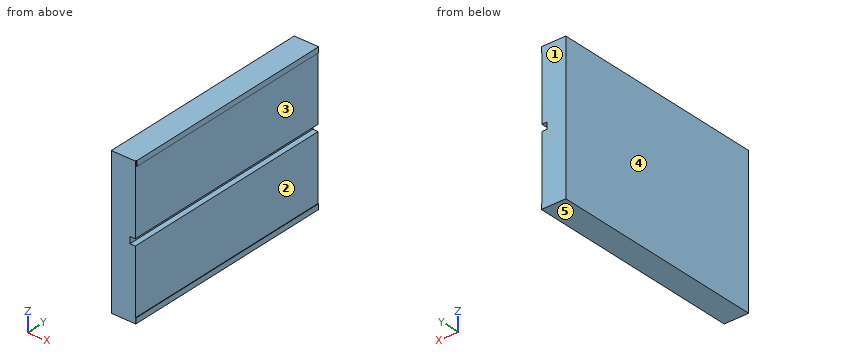
from build123d import *

# Parameters (mm, degrees)
SKETCH1_W           = 9
SKETCH1_H           = 55
BOSS_EXTRUDE1_DEPTH = 82
SKETCH2_W           = 1.230757027
SKETCH2_H           = 82
CUT_EXTRUDE1_DEPTH  = 2
SKETCH3_W           = 2
SKETCH3_H           = 81.454636245
SKETCH3_H_2         = 81.981396298
BOSS_EXTRUDE2_DEPTH = 0.2


with BuildPart() as part:
    # Sketch1 → Boss-Extrude1 (new body)
    with BuildSketch(Plane(origin=(0, 0, 0), x_dir=(1, 0, 0), z_dir=(0, 1, 0))):
        Rectangle(SKETCH1_W, SKETCH1_H)
    extrude(amount=BOSS_EXTRUDE1_DEPTH)

    # Sketch2 → Cut-Extrude1 (cut)
    with BuildSketch(Plane(origin=(4.5, 0, 0), x_dir=(0, 0, -1), z_dir=(1, 0, 0))):
        with Locations((-0.615378514, 41)):
            Rectangle(SKETCH2_W, SKETCH2_H)
        with Locations((0.615378514, 41)):
            Rectangle(SKETCH2_W, SKETCH2_H)
    extrude(amount=-CUT_EXTRUDE1_DEPTH, mode=Mode.SUBTRACT)

    # Sketch3 → Boss-Extrude2 (add)
    with BuildSketch(Plane(origin=(4.5, 0, 0), x_dir=(0, 0, -1), z_dir=(1, 0, 0))):
        with Locations((-26.5, 41.272681877)):
            Rectangle(SKETCH3_W, SKETCH3_H)
        with Locations((26.5, 41.009301851)):
            Rectangle(SKETCH3_W, SKETCH3_H_2)
    extrude(amount=BOSS_EXTRUDE2_DEPTH)


solid = part.part
Geometry: final body of the model. Coordinates: model frame, mm. Face numbers are marked on the shaded views. A direction names the side the tool comes from. Round coordinates to 2 decimals unless told otherwise and drop trailing zeros. Order: outer loops, then holes, each group sorted by start corner. A loop starts at its lowest first (then second) coordinate and runs counter-clockwise, first axis right, second up. Notation, with made-up numbers: (-31, 5) - (-1, 5) arc R24 ccw to (-1, 36) - close; hole circle Ø2 at (17, -7). An arc over 180 degrees is marked (long way). Write each question's results on one line, items separated by ' | '.
Item 1: Section B-B, the plane z = 19.5. Return the cut outline in (x, y).
Completed:
outline: (-4.5, 0) - (4.5, 0) - (4.5, 82) - (-4.5, 82) - close
Item 2: First-contact query: pin 1 Ø5 at (y, z) = (72.5, 1.5) entering from +X; pin 2 Ø1.2 at (y, z) = (39.5, 0) entering from +X. Flat tips, straight axial feed; report the tip coordinate or a pass-through.
Completed:
pin 1: x = 4.5 | pin 2: x = 2.5
Item 3: Material intervals for line 1 along Z through (x, y) = (4, 23); line 2 along X through (y, z) = (6, -9), sorted ascending. Write a range as [from, to].
Completed:
line 1: [-27.5, -1.23], [1.23, 27.5] | line 2: [-4.5, 4.5]
Item 4: Section A-A, the plane y = 56.5. Return the cut outline in (x, z), and give its area (3 significant figures).
Completed:
outline: (-4.5, -27.5) - (4.7, -27.5) - (4.7, -25.5) - (4.5, -25.5) - (4.5, -1.23) - (2.5, -1.23) - (2.5, 1.23) - (4.5, 1.23) - (4.5, 25.5) - (4.7, 25.5) - (4.7, 27.5) - (-4.5, 27.5) - close | area: 491 mm^2
Item 5: Mould query, pull axis Z, two halves, no side actions, for the marked faces 3, 4 and 5. Classes: pulls with the +Z half, pulls with the -Z half, needs draft (parallel to the pull), parting line crosses it, or undercut.
Completed:
face 3: undercut | face 4: needs draft | face 5: pulls with the -Z half
Item 6: Reachability of the marked faces 1 and 2 from +Z, -Z, +X, -X, +Y, -Y: full face, straight path, thin tool, end or side. Return the list, or none.
Completed:
face 1: +Z, -Z, +X, -X, +Y | face 2: +X, +Y, -Y
